The drawing under review shows one solid part. Ordinate dimensions are in mm from its lowest x, y, z. A direction names the side the tool comes from. Coordinates: 2 decimals unless noted, no trailing zeros. Order: outer loops, then holes, each group sorted by start corner. A loop starts at its lowest first (then second) coordinate and runs counter-clockwise, first axis right, second up.
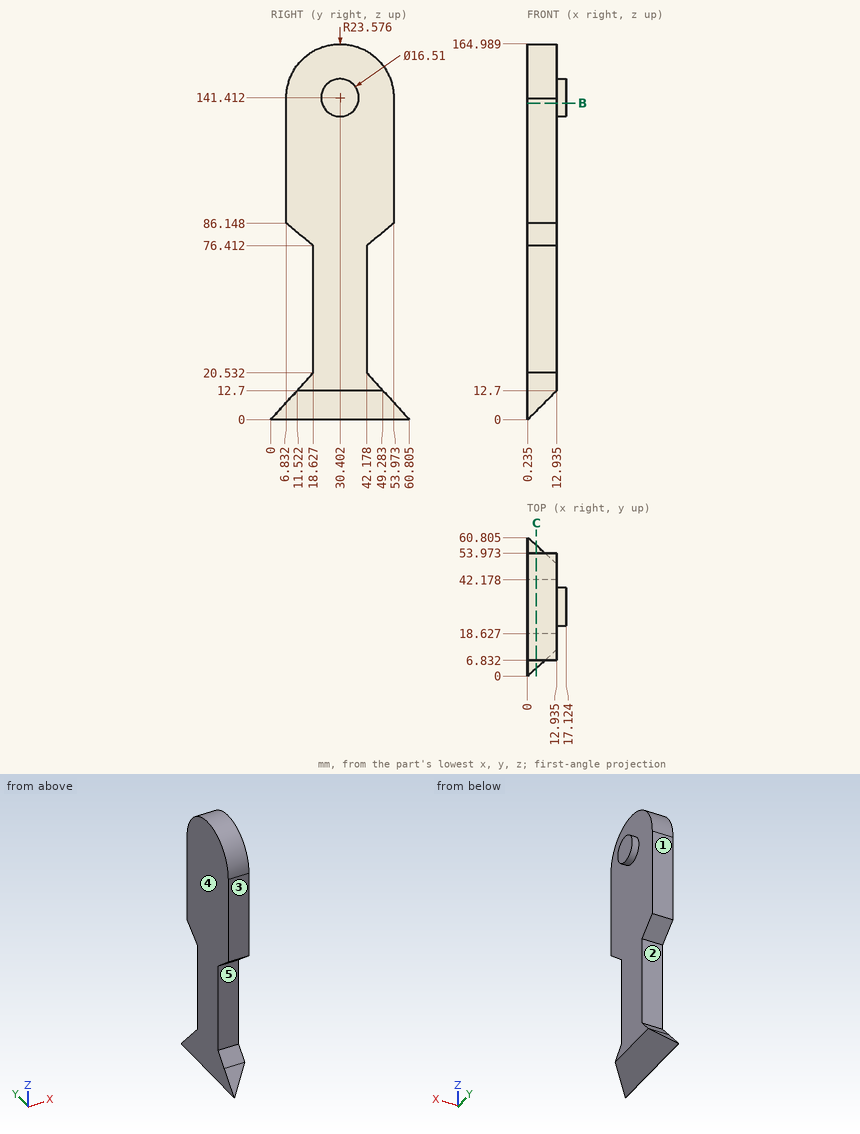
(1) Wall thickness on probe 1 along X at (y, z) = (21, 53.5) (1 decimal); probe 2 along Y at (x, z) = (8.5, 115); probe 3 along Y at (x, z) = (10.5, 51.5): over which ranges is each line inside the solid? List them lowest first.
A:
probe 1: x = 0 to 12.9
probe 2: y = 6.83 to 53.97
probe 3: y = 18.63 to 42.18
(2) For pin 1 Ø12 at (y, z) = (23, 98) entering from +X (1 decimal); pin 2 Ø6 at (x, y) = (9.5, 43) entering from +Z; pin 3 Ø1 at (x, y) = (12, 22.5) entering from -Z (1 decimal), all flat-tipped, find the tip position at first contact; note any pin that passes through.
A:
pin 1: stops at x = 12.9
pin 2: stops at z = 162.95
pin 3: stops at z = 11.3
(3) Machinability: for the marked faces 1, 2, 3, 4 and 5, which of the approach directions +Z, -Z, +X, -X, +Y, -Y give a long, thin tool a straight path to every point of the face, cutting with its end or side? Answer none if there is none.
A:
face 1: +Z, +X, -X, +Y
face 2: +X, -X, +Y
face 3: +Z, +X, -X, -Y
face 4: +Z, -Z, -X, +Y, -Y
face 5: +X, -X, -Y
(4) We need section C-C, the plane x = 4. Write out the cut boundary in (y, z) (1 decimal).
A:
outline: (3.4, 3.8) - (57.4, 3.8) - (42.2, 20.5) - (42.2, 76.4) - (54, 86.1) - (54, 140.9) arc R23.6 ccw (long way) to (6.8, 140.9) - (6.8, 86.1) - (18.6, 76.4) - (18.6, 20.5) - close
(5) We need section B-B, the plane z = 139. Write out the cut boundary in (x, y) (1 decimal), and give its area (3 significant figures).
A:
outline: (0, 6.8) - (12.9, 6.8) - (12.9, 22.5) - (17.1, 22.5) - (17.1, 38.3) - (12.9, 38.3) - (12.9, 54) - (0, 54) - close
area: 676 mm2
